Part model, mm, in its own coordinate system. A direction names the side the tool comes from. Give positions to 0.01 mm unless a question says otherwise; leave off trailing zeros. Write each loop counter-clockwise with the first axis right and the second up, starting at its lowest first coordinate (ties: lowest second). Pieces come first, ordered by that corner, then holes.
```python
from build123d import *

# Parameters (mm, degrees)
F1_DEPTH = 25.4
F2_W     = 25.4
F2_H     = 25.4
F3_DEPTH = 25.4


with BuildPart() as f1:
    # F0 (on Top) → F1 (new body)
    with BuildSketch(Plane.XY):
        Polygon((0, -12.7), (25.4, -12.7), (25.4, 12.7), (-25.4, 12.7), (-25.4, -12.7), (-25.4, -38.1), (0, -38.1), align=None)
    extrude(amount=F1_DEPTH)

    # F2 (on face) → F3 (join)
    with BuildSketch(Plane.XY.offset(25.4)):
        with Locations((-12.7, 0)):
            Rectangle(F2_W, F2_H)
    extrude(amount=F3_DEPTH)


solid = f1.part
```
1) Saw through at D-D, the plane z = 45. Write the cut outline in (x, y), then the cut area to 3 significant figures.
Answers follow:
outline: (-25.4, -12.7) - (0, -12.7) - (0, 12.7) - (-25.4, 12.7) - close
area: 645 mm2
2) 3-axis set-ups, long thin cutter, end or side, ignore diameter. For faces 1 (the face through (13, 0, 25.4)), 2 (the face through (-13, -25, 25.4)), 3 (the face through (0, -26, 13)): which of +Z, -Z, +X, -X, +Y, -Y reach the whole face in a straight line?
Answers follow:
face 1: +Z, +X, +Y, -Y
face 2: +Z, +X, -X, -Y
face 3: +Z, -Z, +X, -Y
3) Saw through at B-B, the plane z = 19. Write the cut outline in (x, y).
Answers follow:
outline: (-25.4, -38.1) - (0, -38.1) - (0, -12.7) - (25.4, -12.7) - (25.4, 12.7) - (-25.4, 12.7) - close
4) Saw through at A-A, the plane y = 5.5. Write the cut outline in (x, z).
Answers follow:
outline: (-25.4, 0) - (25.4, 0) - (25.4, 25.4) - (0, 25.4) - (0, 50.8) - (-25.4, 50.8) - close
5) Wall check: L1, parallel to Y at x = -1.5, z = 30; L2, parallel to X at y = -24.5, z = 14.5; L3, parallel to Z at x = -12.5, y = -20.5. Give the ranges that are in metal, low to high.
Answers follow:
L1: y = -12.7 to 12.7
L2: x = -25.4 to 0
L3: z = 0 to 25.4
6) Pin check, flat tips, straight feed: pin 1 Ø5 at (x, y) = (-16.5, -6.5) entering from -Z; pin 2 Ø20.5 at (y, z) = (-2.5, 42.5) entering from +X; pin 3 Ø7.5 at (x, z) = (-12, 41.5) entering from -Y. Stop position of each tip, or through.
Answers follow:
pin 1: stops at z = 0
pin 2: stops at x = 0
pin 3: stops at y = -12.7
7) Saw through at C-C, the plane x = 4. Write the cut outline in (y, z).
Answers follow:
outline: (-12.7, 0) - (12.7, 0) - (12.7, 25.4) - (-12.7, 25.4) - close
